Source: CAD feature listing. Evaluate the final solid. Frame: model axes, mm. Give positions to 0.01 mm unless a question says otherwise; leave off trailing zeros. Order: outer loops, then holes, each group sorted by start corner. A loop starts at its lowest first (then second) coordinate and runs counter-clockwise, first axis right, second up. Notation, with made-up numbers: M -0.5,0 L 31.5,0 A19 ccw 31.5,25 Z; hole C 87,42 d3. An arc over 180 degrees is marked long. Answer as a JSON object with one key per item and string values. Group by question number.
1. Pin query (flat end, axial travel): P1, Ø1.5, axis at x = -26.84, y = 17.43, coming from the +Z side. Return the tip coordinate at first contact, or that it passes through.
2. Section query A-A (x = 0). Output: boundary loops of the cut face in (y, z).
3. Pull-direction query (Y, two-part tool) for faces 1 (the flat face through (0, -23, 1.55)), 2 (the cylindrical face through (-28, -21, 1)); classes: +Y half, -Y half, draft (parallel to the pull), parting line (faces both ways), or undercut.
4. Section query D-D (y = 23). Output: boundary loops of the cut face in (x, z), plus the area to 3 significant figures.
5. Section query B-B (z = 1). Output: boundary loops of the cut face in (x, y), plus the area to 3 significant figures.
6. Section query C-C (x = -15). Output: boundary loops of the cut face in (y, z), plus the area to 3 significant figures.
7. Material intervals for L1, parallel to Y at x = -0.5, z = 1.25; L2, parallel to X at y = 13, z = 1.2; L3, parallel to X at y = -12, z = 0.85, sorted ascending. Write a range as [from, to].
from build123d import *

# Parameters (mm, degrees)
SKETCH1_R           = 35
BOSS_EXTRUDE1_DEPTH = 1.3
SKETCH2_R           = 22
CUT_EXTRUDE1_DEPTH  = 50.514543318
MOVE_FACE1_BY       = 0.7
SKETCH5_R           = 0.95
CUT_EXTRUDE4_DEPTH  = 50.501111099
CIRPATTERN2_COUNT   = 5
MOVE_FACE2_BY       = 0.25


with BuildPart() as part:
    # Sketch1 → Boss-Extrude1 (new body)
    with BuildSketch(Plane.XY):
        Circle(SKETCH1_R)
    extrude(amount=BOSS_EXTRUDE1_DEPTH)

    # Sketch2 → Cut-Extrude1 (cut, through all)
    with BuildSketch(Plane.XY.offset(1.3)):
        Circle(SKETCH2_R)
    extrude(amount=-CUT_EXTRUDE1_DEPTH, mode=Mode.SUBTRACT)

    # Move Face1: a face moved inward by 0.7
    extrude(part.faces().sort_by_distance((0, -28, 0))[0], amount=MOVE_FACE1_BY, dir=(0, 0, 1), mode=Mode.SUBTRACT)

    # Sketch5 → Cut-Extrude4 (cut, through all)
    with BuildSketch(Plane.XY.offset(1.3)):
        with Locations((8.282209443, 30.909626441)):
            Circle(SKETCH5_R)
    cut_extrude4 = extrude(amount=-CUT_EXTRUDE4_DEPTH, mode=Mode.SUBTRACT)

    # CirPattern2: Cut-Extrude4 ×5 about axis
    cirpattern2_axis = Axis((0, 0, 0), (0, 0, 1))
    for i in range(1, CIRPATTERN2_COUNT):
        add(cut_extrude4.rotate(cirpattern2_axis, i * 360 / CIRPATTERN2_COUNT), mode=Mode.SUBTRACT)

    # Move Face2: a face moved outward by 0.25
    extrude(part.faces().sort_by_distance((0, -28, 1.3))[0], amount=MOVE_FACE2_BY, dir=(0, 0, 1))


solid = part.part
Answer sheet:
{
 "1": {"P1": "through"},
 "2": {"outline": "M -35,0.7 L -22,0.7 L -22,1.55 L -35,1.55 Z; M 22,0.7 L 35,0.7 L 35,1.55 L 22,1.55 Z"},
 "3": {"face 1": "draft", "face 2": "parting line"},
 "4": {"outline": "M -26.38,0.7 L 26.38,0.7 L 26.38,1.55 L -26.38,1.55 Z", "area": "44.8 mm^2"},
 "5": {"outline": "C 0,0 d70; hole C -26.84,17.43 d1.9; hole C -24.87,-20.14 d1.9; hole C 0,0 d44; hole C 8.28,30.91 d1.9; hole C 11.47,-29.87 d1.9; hole C 31.96,1.67 d1.9", "area": "2,310 mm^2"},
 "6": {"outline": "M -31.62,0.7 L -16.09,0.7 L -16.09,1.55 L -31.62,1.55 Z; M 16.09,0.7 L 31.62,0.7 L 31.62,1.55 L 16.09,1.55 Z", "area": "26.4 mm^2"},
 "7": {"L1": "[-35, -21.99], [21.99, 35]", "L2": "[-32.5, -17.75], [17.75, 32.5]", "L3": "[-32.88, -18.44], [18.44, 32.88]"}
}
